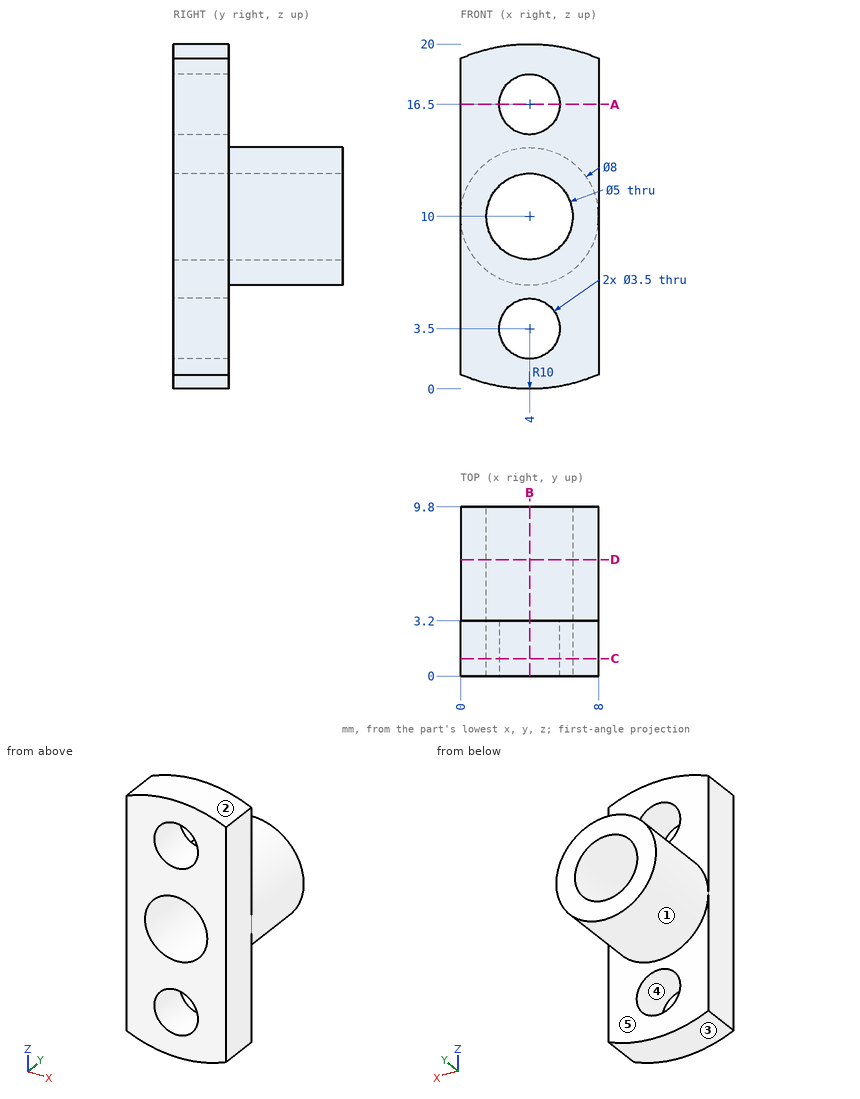
Source: three-view drawing plus pictorial views. Frame: mm from the lowest corner of the part. A direction names the side the tool comes from. Give positions to 0.01 mm unless a question says otherwise; leave off trailing zeros. Order: outer loops, then holes, each group sorted by start corner. A loop starts at its lowest first (then second) coordinate and runs counter-clockwise, first axis right, second up. Notation, with made-up numbers: (-31, -38) - (18, -38) arc R21 ccw to (18, -22) - close; hole circle Ø10 at (71, -26.75). An arc over 180 degrees is marked (long way). Answer as a JSON object with one key per item and string values. Group by question number.
Q1. Mould query, pull axis X, two halves, no side actions, for the marked faces 3, 4 and 5. Classes: pulls with the +X half, pulls with the -X half, needs draft (parallel to the pull), parting line crosses it, or undercut.
Q2. Cut plane B-B, the plane x = 4. Output: boundary loops of the cut face in (y, z), then the cut area to 3 significant figures.
Q3. Cut plane C-C, the plane y = 1. Output: boundary loops of the cut face in (x, z), then the cut area to 3 significant figures.
Q4. Set-up query: the marked faces 1 and 2. Return all of +Z, -Z, +X, -X, +Y, -Y with unobstructed straight access to the full face (end or side cutting, diameter ignored); none if empty.
Q5. Cut plane A-A, the plane z = 16.5. Output: boundary loops of the cut face in (x, y).
Q6. Cut plane D-D, the plane y = 6.75. Output: boundary loops of the cut face in (x, z).
Q7. First-contact query: pin 1 Ø2 at (x, z) = (4, 3.5) entering from -Y; pin 2 Ø3 at (y, z) = (5.5, 8) entering from +X. Flat tips, straight axial feed; report the tip coordinate or a pass-through.
Q8. Line query: probe 1 along X at (y, z) = (0.7, 3.5); probe 2 along Z at (x, y) = (4, 6.75); probe 3 along X at (y, z) = (3.25, 10). Output: solid intervals per line, ascending.
Results:
{
 "1": {"face 3": "parting line crosses it", "face 4": "undercut", "face 5": "needs draft"},
 "2": {"outline": "(0, 0) - (3.2, 0) - (3.2, 1.75) - (0, 1.75) - close; (0, 5.25) - (3.2, 5.25) - (3.2, 6) - (9.8, 6) - (9.8, 7.5) - (0, 7.5) - close; (0, 12.5) - (9.8, 12.5) - (9.8, 14) - (3.2, 14) - (3.2, 14.75) - (0, 14.75) - close; (0, 18.25) - (3.2, 18.25) - (3.2, 20) - (0, 20) - close", "area": "45.4 mm^2"},
 "3": {"outline": "(0, 0.83) arc R10 ccw to (8, 0.83) - (8, 19.17) arc R10 ccw to (0, 19.17) - close; hole circle Ø5 at (4, 10); hole circle Ø3.5 at (4, 3.5); hole circle Ø3.5 at (4, 16.5)", "area": "117 mm^2"},
 "4": {"face 1": "+Y", "face 2": "+Z, +Y, -Y"},
 "5": {"outline": "(0, 0) - (2.25, 0) - (2.25, 3.2) - (0, 3.2) - close; (5.75, 0) - (8, 0) - (8, 3.2) - (5.75, 3.2) - close"},
 "6": {"outline": "circle Ø8 at (4, 10); hole circle Ø5 at (4, 10)"},
 "7": {"pin 1": "through", "pin 2": "x = 7.97"},
 "8": {"probe 1": "0 to 2.25, 5.75 to 8", "probe 2": "6 to 7.5, 12.5 to 14", "probe 3": "0 to 1.5, 6.5 to 8"}
}
